Geometry: see drawing. Coordinates: mm, zero at the bounding-box minimum. A direction names the side the tool comes from. Coordinates: 2 decimals unless noted, no trailing zeros. Loops run counter-clockwise (first coordinate to the right, second up) from the corner with the lowest first, then second, coordinate; pieces in that order, holes last. Notation, with made-up numbers: (-39.75, 10) -> (-13.75, 10) arc R13 ccw to (-13.75, 24) -> close; hole circle Ø2 at (34, 52.5). An arc over 180 degrees is marked (long way). One line per item, written item: value. Start each with the question number.
Item 1: Section query C-C on z = 13.75. Return loops of the section in (x, y).
Item 2: Ray query, probe 1 along Y at (x, z) = (37.4, 3.05); probe 2 along Y at (x, z) = (61, 6) (1 decimal); probe 3 along X at (y, z) = (27, 5.5) (1 decimal). Return the intervals inside material, ascending. Write a range as from..to.
Item 3: Section query B-B on x = 37.4. Give the number of separate pieces and of enclosed holes in the cut face, then the cut area to 3 significant figures.
Item 4: Section query D-D on z = 19.5. Return loops of the section in (x, y).
Item 5: Contact query for flat-ended pins moving along their axis: pin 1 Ø2.5 at (x, y) = (12.64, 57.15) entering from -Z; pin 2 Ø10 at (x, z) = (34.5, 12) entering from -Y; pin 3 Ø1.3 at (x, y) = (51.14, 8.87) entering from -Z; pin 4 Ø3 at (x, y) = (12.64, 17.65) entering from +Z. Output: stop coordinate, or through.
Item 6: Section query A-A on y = 37.4. Return loops of the section in (x, z).
Item 7: Set-up query: the marked faces 3 and 4. Return all of +Z, -Z, +X, -X, +Y, -Y with unobstructed straight access to the full face (end or side cutting, diameter ignored); none if empty.
Item 8: Mould query, pull axis X, two halves, no side actions, for the marked faces 1 and 2. Classes: +X half, -X half, draft (parallel to the pull), parting line (faces both ways), or undercut.
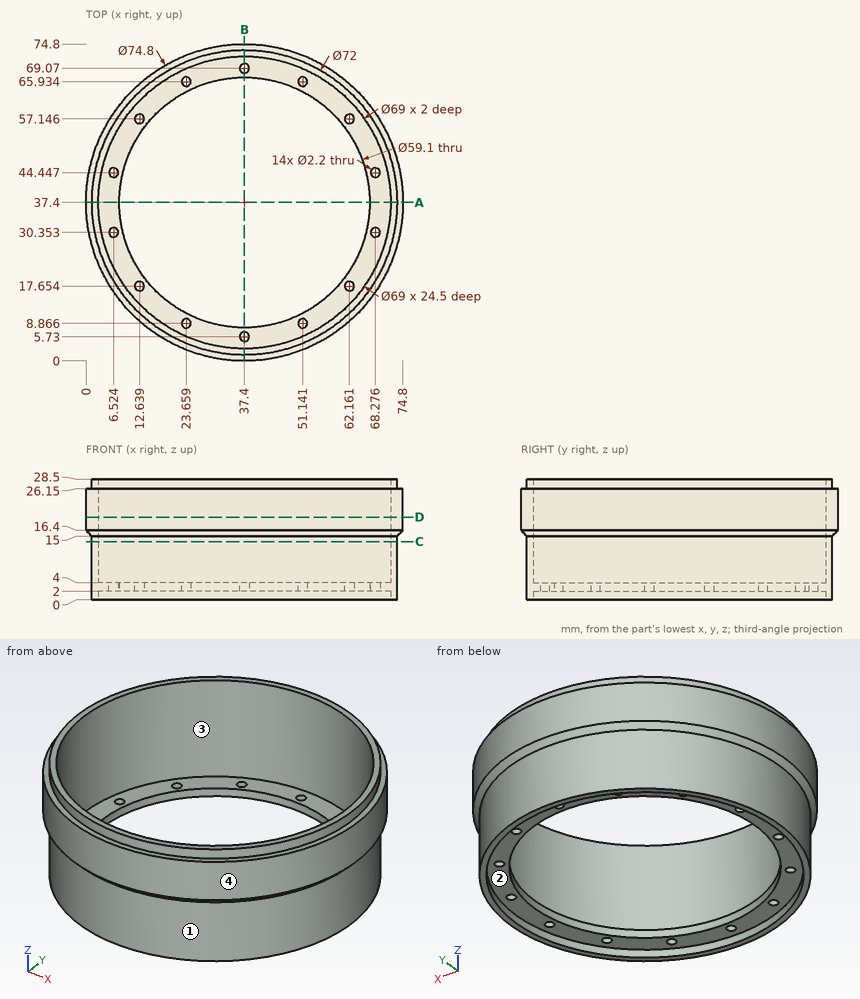
Reply:
1. outline: circle Ø72 at (37.4, 37.4); hole circle Ø69 at (37.4, 37.4)
2. probe 1: y = 1.4..4.63, 6.83..7.85, 66.95..67.97, 70.17..73.4
2. probe 2: y = 10.2..12.2, 62.6..64.6
2. probe 3: x = 2.9..4.5, 70.3..71.9
3. separate pieces: 4
3. enclosed holes: 0
3. area: 126 mm²
4. outline: circle Ø74.8 at (37.4, 37.4); hole circle Ø69 at (37.4, 37.4)
5. pin 1: stops at z = 2
5. pin 2: stops at y = 0
5. pin 3: passes through
5. pin 4: stops at z = 4
6. outline: (0, 16.4) -> (1.4, 15) -> (1.4, 0) -> (2.9, 0) -> (2.9, 2) -> (7.85, 2) -> (7.85, 4) -> (2.9, 4) -> (2.9, 28.5) -> (1.4, 28.5) -> (1.4, 26.15) -> (0, 26.15) -> close; (66.95, 2) -> (71.9, 2) -> (71.9, 0) -> (73.4, 0) -> (73.4, 15) -> (74.8, 16.4) -> (74.8, 26.15) -> (73.4, 26.15) -> (73.4, 28.5) -> (71.9, 28.5) -> (71.9, 4) -> (66.95, 4) -> close
7. face 3: +Z
7. face 4: +Z, -Z
8. face 1: parting line
8. face 2: undercut
